Part print with two shaded views. Sizes in mm from the minimum x, y, z corner. Coordinates: 2 decimals unless noted, no trailing zeros. Loops run counter-clockwise (first coordinate to the right, second up) from the corner with the lowest first, then second, coordinate; pieces in that order, holes last. Notation, with made-up numbers: (1.25, 37) -> (30.25, 37) arc R31 cw to (30.25, 70) -> close; hole circle Ø6 at (12, 88.5). An arc over 180 degrees is marked (long way). Return JSON: item names as keys, results as strings. Group by question number.
(1) Flat gauge pin, fed straight in: pin 1 Ø8 at (x, y) = (26, 15) entering from -Z. Where does the tip first touch, or does it go through?
(2) Saw through at D-D on y = 58. Write the cut outline in (x, z), then the cut area to 3 significant figures.
(3) Saw through at A-A on y = 10. Write the cut outline in (x, z), then the cut area to 3 significant figures.
(4) Saw through at B-B on x = 24. Write the cut outline in (y, z), then the cut area to 4 significant figures.
(5) Saw through at C-C on z = 0.75. Write the cut outline in (x, y), then the cut area to 3 significant figures.
(6) Probe L1, parallel to X at y = 10, z = 1.8; L2, parallel to Y at x = 24.5, z = 1.05; L3, parallel to X at y = 57.5, z = 0.6. List the from-to ranges inside material, lowest first.
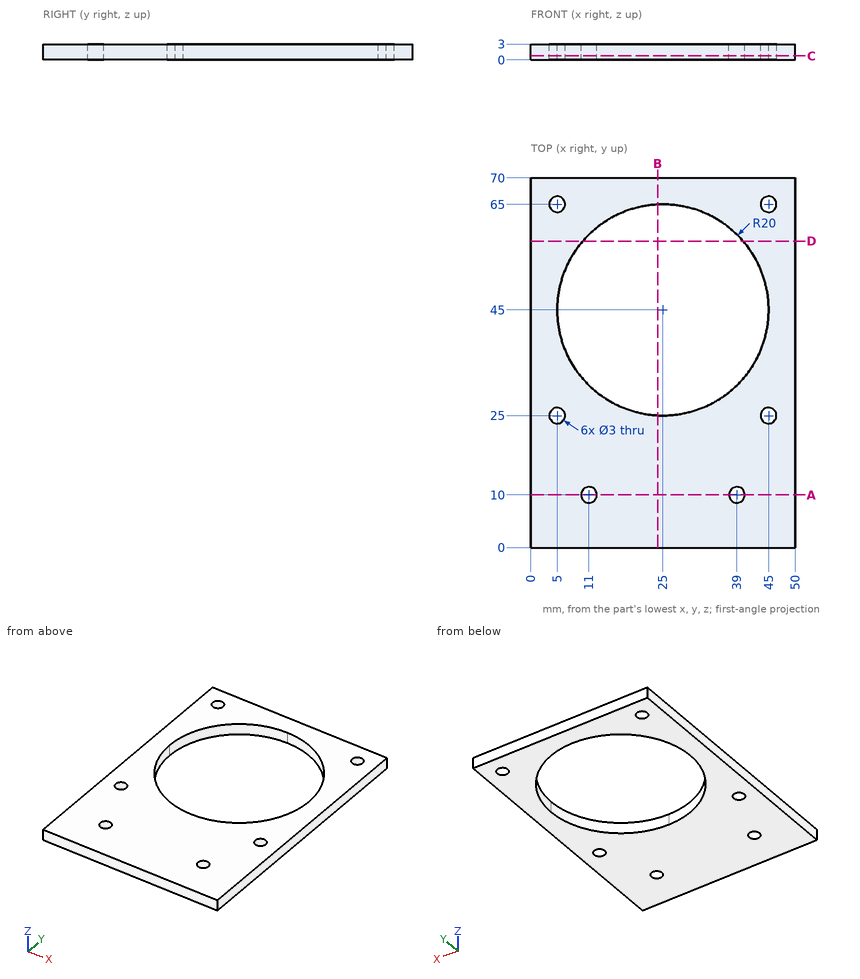
Geometry results:
{
 "1": {"pin 1": "z = 0"},
 "2": {"outline": "(0, 0) -> (9.8, 0) -> (9.8, 3) -> (0, 3) -> close; (40.2, 0) -> (50, 0) -> (50, 3) -> (40.2, 3) -> close", "area": "58.8 mm²"},
 "3": {"outline": "(0, 0) -> (9.5, 0) -> (9.5, 3) -> (0, 3) -> close; (12.5, 0) -> (37.5, 0) -> (37.5, 3) -> (12.5, 3) -> close; (40.5, 0) -> (50, 0) -> (50, 3) -> (40.5, 3) -> close", "area": "132 mm²"},
 "4": {"outline": "(0, 0) -> (25.03, 0) -> (25.03, 3) -> (0, 3) -> close; (64.97, 0) -> (70, 0) -> (70, 3) -> (64.97, 3) -> close", "area": "90.15 mm²"},
 "5": {"outline": "(0, 0) -> (50, 0) -> (50, 70) -> (0, 70) -> close; hole circle Ø3 at (5, 25); hole circle Ø3 at (5, 65); hole circle Ø40 at (25, 45); hole circle Ø3 at (11, 10); hole circle Ø3 at (39, 10); hole circle Ø3 at (45, 25); hole circle Ø3 at (45, 65)", "area": "2,200 mm²"},
 "6": {"L1": "0 to 9.5, 12.5 to 37.5, 40.5 to 50", "L2": "0 to 25.01, 64.99 to 70", "L3": "0 to 9.39, 40.61 to 50"}
}
